CAD build for the part. Positions are in the model's coordinates, mm. A direction names the side the tool comes from. Round coordinates to 2 decimals unless told otherwise and drop trailing zeros. Loops run counter-clockwise (first coordinate to the right, second up) from the corner with the lowest first, then second, coordinate; pieces in that order, holes last.
```python
from build123d import *

# Parameters (mm, degrees)
BODY_DEPTH                            = 45
MOUNTING_HOLES_REACH                  = 17
SKETCH3_R                             = 4.3
SKETCH3_R_2                           = 1.5
MOUNTING_HOLE_COUNTERBORE_DEPTH       = 3.5
STRESS_CONCENTRATION_RELIEF_FILLETS_R = 10
SLOT_DEPTH                            = 72.568542495


with BuildPart() as part:
    # Sketch1 → Body (new body)
    with BuildSketch(Plane(origin=(0, 0, 0), x_dir=(1, 0, 0), z_dir=(0, 1, 0))):
        Polygon((0, 0), (0, 101.213203436), (56.568542495, 157.781745931), (56.568542495, 202.781745931), (71.568542495, 202.781745931), (71.568542495, 151.568542495), (15, 95), (15, 0), align=None)
    extrude(amount=BODY_DEPTH)

    # Sketch3 → Mounting Holes (cut, up to next)
    with BuildSketch(Plane.ZY.offset(-56.568542495), mode=Mode.PRIVATE) as mounting_holes_sk1:
        with Locations((-180.281745931, 22.5)):
            Circle(SKETCH3_R)
    mounting_holes_tool1 = extrude(mounting_holes_sk1.sketch, amount=-MOUNTING_HOLES_REACH, mode=Mode.PRIVATE) & part.part
    add(mounting_holes_tool1.solids().sort_by_distance((56.568542, 22.5, -180.281746))[0], mode=Mode.SUBTRACT)
    # Sketch3 → Mounting Holes (cut, up to next)
    with BuildSketch(Plane.ZY.offset(-56.568542495), mode=Mode.PRIVATE) as mounting_holes_sk2:
        with Locations((-180.281745931, 37.5)):
            Circle(SKETCH3_R_2)
    mounting_holes_tool2 = extrude(mounting_holes_sk2.sketch, amount=-MOUNTING_HOLES_REACH, mode=Mode.PRIVATE) & part.part
    add(mounting_holes_tool2.solids().sort_by_distance((56.568542, 37.5, -180.281746))[0], mode=Mode.SUBTRACT)
    # Sketch3 → Mounting Holes (cut, up to next)
    with BuildSketch(Plane.ZY.offset(-56.568542495), mode=Mode.PRIVATE) as mounting_holes_sk3:
        with Locations((-165.281745931, 22.5)):
            Circle(SKETCH3_R_2)
    mounting_holes_tool3 = extrude(mounting_holes_sk3.sketch, amount=-MOUNTING_HOLES_REACH, mode=Mode.PRIVATE) & part.part
    add(mounting_holes_tool3.solids().sort_by_distance((56.568542, 22.5, -165.281746))[0], mode=Mode.SUBTRACT)
    # Sketch3 → Mounting Holes (cut, up to next)
    with BuildSketch(Plane.ZY.offset(-56.568542495), mode=Mode.PRIVATE) as mounting_holes_sk4:
        with Locations((-180.281745931, 7.5)):
            Circle(SKETCH3_R_2)
    mounting_holes_tool4 = extrude(mounting_holes_sk4.sketch, amount=-MOUNTING_HOLES_REACH, mode=Mode.PRIVATE) & part.part
    add(mounting_holes_tool4.solids().sort_by_distance((56.568542, 7.5, -180.281746))[0], mode=Mode.SUBTRACT)
    # Sketch3 → Mounting Holes (cut, up to next)
    with BuildSketch(Plane.ZY.offset(-56.568542495), mode=Mode.PRIVATE) as mounting_holes_sk5:
        with Locations((-195.281745931, 22.5)):
            Circle(SKETCH3_R_2)
    mounting_holes_tool5 = extrude(mounting_holes_sk5.sketch, amount=-MOUNTING_HOLES_REACH, mode=Mode.PRIVATE) & part.part
    add(mounting_holes_tool5.solids().sort_by_distance((56.568542, 22.5, -195.281746))[0], mode=Mode.SUBTRACT)

    # Sketch4 → Mounting Hole Counterbore (cut)
    with BuildSketch(Plane.ZY.offset(-56.568542495)):
        Polygon((-162.431745931, 20.854551733), (-162.431745931, 24.145448267), (-165.281745931, 25.790896534), (-168.131745931, 24.145448267), (-168.131745931, 20.854551733), (-165.281745931, 19.209103466), align=None)
        Polygon((-178.636297663, 40.35), (-181.927194198, 40.35), (-183.572642465, 37.5), (-181.927194198, 34.65), (-178.636297663, 34.65), (-176.990849396, 37.5), align=None)
        Polygon((-181.927194198, 4.65), (-178.636297663, 4.65), (-176.990849396, 7.5), (-178.636297663, 10.35), (-181.927194198, 10.35), (-183.572642465, 7.5), align=None)
        Polygon((-198.131745931, 24.145448267), (-198.131745931, 20.854551733), (-195.281745931, 19.209103466), (-192.431745931, 20.854551733), (-192.431745931, 24.145448267), (-195.281745931, 25.790896534), align=None)
    extrude(amount=-MOUNTING_HOLE_COUNTERBORE_DEPTH, mode=Mode.SUBTRACT)

    # Stress Concentration Relief Fillets
    stress_concentration_relief_fillets_edges = [part.edges().sort_by_distance(p)[0] for p in [
        (0, 22.5, -101.213203436),
        (56.568542495, 22.5, -157.781745931),
        (71.568542495, 22.5, -151.568542495),
        (15, 22.5, -95),
    ]]
    fillet(stress_concentration_relief_fillets_edges, radius=STRESS_CONCENTRATION_RELIEF_FILLETS_R)

    # Sketch5 → Slot (cut, through all)
    with BuildSketch(Plane.ZY):
        with BuildLine():
            Line((-72.071067812, 26.8), (-15, 26.8))
            ThreePointArc((-15, 26.8), (-10.7, 22.5), (-15, 18.2))
            Line((-15, 18.2), (-72.071067812, 18.2))
            ThreePointArc((-72.071067812, 18.2), (-76.371067812, 22.5), (-72.071067812, 26.8))
        make_face()
    extrude(amount=-SLOT_DEPTH, mode=Mode.SUBTRACT)


solid = part.part
```
Item 1: 3-axis set-ups, long thin cutter, end or side, ignore diameter. For faces 1 (the flat face through (15, 17, -46)), 2 (the flat face through (64, 22, -202.782)), 3 (the flat face through (56.569, 22, -187)), 4 (the cylindrical face through (7.4, 22.41, -76.37)), 5 (the flat face through (60.069, 39, -181)): which of +Z, -Z, +X, -X, +Y, -Y reach the whole face in a straight line?
Answers follow:
face 1: +Z, +X, +Y, -Y
face 2: -Z, +X, -X, +Y, -Y
face 3: -Z, -X, +Y, -Y
face 4: +X, -X
face 5: -X
Item 2: Cut at A-A, the plane y = 14.5. Give the cut face in (x, z).
Answers follow:
outline: (0, -97.07) arc R10 ccw to (2.93, -104.14) - (53.64, -154.85) arc R10 cw to (56.57, -161.92) - (56.57, -202.78) - (71.57, -202.78) - (71.57, -155.71) arc R10 ccw to (68.64, -148.64) - (17.93, -97.93) arc R10 cw to (15, -90.86) - (15, 0) - (0, 0) - close
Item 3: Cut at B-B, the plane x = 65. Give the cut face in (y, z), plus the area to 3 significant figures.
Answers follow:
outline: (0, -202.78) - (45, -202.78) - (45, -145) - (0, -145) - close; hole circle Ø3 at (7.5, -180.28); hole circle Ø8.6 at (22.5, -180.28); hole circle Ø3 at (22.5, -195.28); hole circle Ø3 at (22.5, -165.28); hole circle Ø3 at (37.5, -180.28)
area: 2,510 mm2
Item 4: Probe line 1 (Y direction, x = 62, z = -183); line 2 (Z direction, x = 65, y = 22); line 3 (Z direction, x = 62, y = 22). List the from-to ranges inside material, lowest first.
Answers follow:
line 1: y = 0 to 19.17, 25.83 to 45
line 2: z = -202.78 to -196.7, -193.87 to -184.55, -176.01 to -166.7, -163.87 to -145
line 3: z = -202.78 to -196.7, -193.87 to -184.55, -176.01 to -166.7, -163.87 to -142
Item 5: Cut at C-C, the plane x = 11.5. Give the cut face in (y, z).
Answers follow:
outline: (0, -112.71) - (45, -112.71) - (45, 0) - (0, 0) - close; hole (18.2, -72.07) arc R4.3 ccw to (26.8, -72.07) - (26.8, -15) arc R4.3 ccw to (18.2, -15) - close
Item 6: Cut at D-D, the plane z = -136.5. Give the cut face in (x, y).
Answers follow:
outline: (35.29, 0) - (56.5, 0) - (56.5, 45) - (35.29, 45) - close
Item 7: Flat gauge pins, fed straight in: P1, Ø1, axis at x = 57.5, y = 22, coming from the +Z side; P2, Ø4, axis at y = 14.5, z = -106, coming from the -X side; P3, Ø3, axis at y = 38, z = -179.5, coming from the -X side. Where does each tip first touch, or does it go through?
Answers follow:
P1: stops at z = -137
P2: stops at x = 2.79
P3: stops at x = 60.07
Item 8: Two-plate mould, pull along Y, no slides. Class faces 6 (the flat face through (25, 0, -109)), 7 (the flat face through (7, 18.2, -43)), 8 (the flat face through (71.569, 17, -180)), 9 (the flat face through (60.069, 21, -166)): released by +Y, released by -Y, zero draft, split by the parting line, or undercut.
Answers follow:
face 6: released by -Y
face 7: undercut
face 8: zero draft
face 9: undercut
